```python
from build123d import *

# Parameters (mm, degrees)
SKETCH1_W           = 23.8
SKETCH1_H           = 9.8
BOSS_EXTRUDE1_DEPTH = 1
SKETCH2_W           = 3
SKETCH2_H           = 6.1
BOSS_EXTRUDE2_DEPTH = 3.25
SKETCH4_W           = 1
SKETCH4_H           = 6.1
BOSS_EXTRUDE3_DEPTH = 1
SKETCH3_R           = 3.3
CUT_EXTRUDE1_DEPTH  = 19.25
FILLET1_R           = 0.2


with BuildPart() as part:
    # Sketch1 → Boss-Extrude1 (new body)
    with BuildSketch(Plane(origin=(0, 0, 0), x_dir=(1, 0, 0), z_dir=(0, 1, 0))):
        with Locations((-11.9, 4.9)):
            Rectangle(SKETCH1_W, SKETCH1_H)
    extrude(amount=BOSS_EXTRUDE1_DEPTH)

    # Sketch2 → Boss-Extrude2 (add)
    with BuildSketch(Plane(origin=(0, 1, 0), x_dir=(1, 0, 0), z_dir=(0, 1, 0))):
        with Locations((-0.5, 5.65)):
            Rectangle(SKETCH2_W, SKETCH2_H)
    extrude(amount=BOSS_EXTRUDE2_DEPTH)

    # Sketch4 → Boss-Extrude3 (add)
    with BuildSketch(Plane.XZ.offset(-1)):
        with Locations((0.5, -5.65)):
            Rectangle(SKETCH4_W, SKETCH4_H)
    extrude(amount=BOSS_EXTRUDE3_DEPTH)

    # Sketch3 → Cut-Extrude1 (cut)
    with BuildSketch(Plane(origin=(1, 0, 0), x_dir=(0, 0, -1), z_dir=(1, 0, 0))):
        with Locations((5.65, 4.25)):
            Circle(SKETCH3_R)
    extrude(amount=-CUT_EXTRUDE1_DEPTH, mode=Mode.SUBTRACT)

    # Fillet1
    fillet1_edges = [part.edges().sort_by_distance(p)[0] for p in [
        (-0.5, 2.990039683, -2.6),
        (-0.5, 2.990039683, -8.7),
    ]]
    fillet(fillet1_edges, radius=FILLET1_R)


solid = part.part
```
Verification items for the finished model (mm, model axes). A direction names the side the tool comes from. Coordinates: 2 decimals unless noted, no trailing zeros. Loops run counter-clockwise (first coordinate to the right, second up) from the corner with the lowest first, then second, coordinate; pieces in that order, holes last. Notation, with made-up numbers: (9.5, -2.5) - (13.5, -2.5) arc R24 cw to (13.5, 20.5) - close; hole circle Ø6 at (87, -9). An arc over 180 degrees is marked (long way). Answer as a JSON object with one key per item and string values.
(1) Scan lines: line 1 along X through (y, z) = (2.35, -8.5); line 2 along Y through (x, z) = (-13.25, -1); line 3 along X through (y, z) = (0.2, -9). Record each from-to range of solid material in increasing order.
Response:
{"line 1": "x = -2 to 1", "line 2": "y = 0 to 1", "line 3": "x = -23.8 to 0"}
(2) Go/stop test with flat-tipped pins: pin 1 Ø1.1 at (y, z) = (2, -8) entering from -X; pin 2 Ø3 at (x, z) = (-15.5, -5) entering from +Y; pin 3 Ø0.8 at (y, z) = (0.5, -1) entering from +X. Record where each tip stops, or that it passes through.
Response:
{"pin 1": "stops at x = -2", "pin 2": "stops at y = 1", "pin 3": "stops at x = 0"}
(3) Cross-section at A-A, the plane y = 1.8. Record the boundary of the cut face in (x, z).
Response:
{"outline": "(-2, -8.7) - (1, -8.7) - (1, -7.86) - (-2, -7.86) - close; (-2, -3.44) - (1, -3.44) - (1, -2.6) - (-2, -2.6) - close"}
(4) Cross-section at D-D, the plane z = -1.75. Record the boundary of the cut face in (x, y), then the cut area to 3 significant figures.
Response:
{"outline": "(-23.8, 0) - (0, 0) - (0, 1) - (-23.8, 1) - close", "area": "23.8 mm²"}
(5) Cross-section at B-B, the plane x = -1. Record the boundary of the cut face in (y, z).
Response:
{"outline": "(0, -9.8) - (1, -9.8) - (1, -8.7) - (2.22, -8.7) arc R0.2 ccw to (2.33, -8.34) arc R3.3 cw to (2.33, -2.96) arc R0.2 ccw to (2.22, -2.6) - (1, -2.6) - (1, 0) - (0, 0) - close"}
(6) Cross-section at C-C, the plane y = 0.6. Record the boundary of the cut face in (x, z), then the cut area to 3 significant figures.
Response:
{"outline": "(-23.8, -9.8) - (0, -9.8) - (0, -8.7) - (1, -8.7) - (1, -2.6) - (0, -2.6) - (0, 0) - (-23.8, 0) - close", "area": "239 mm²"}
(7) Mould release check, pull along Z, two halves, no side actions. Record for faces 6 (the flat face through (-12, 1, -4)), 7 (the cylindrical face through (-5.02, 0.96, -5.4)), 8 (the flat face through (-12.1, 0.5, 0)), 9 (the flat face through (-12.1, 0.5, -9.8)): pulls with the +Z half, pulls with the -Z half, needs draft (parallel to the pull), parting line crosses it, or undercut.
Response:
{"face 6": "needs draft", "face 7": "undercut", "face 8": "pulls with the +Z half", "face 9": "pulls with the -Z half"}
(8) Access from +Z, -Z, +X, -X, +Y, -Y to the whole of each face (thin tool, end or side, straight path). Record for faces 1 (the flat face through (-23.8, 0.5, -4.8)), 2 (the flat face through (1, 0.7, -5.7)), 3 (the flat face through (-2, 1.5, -8)), 4 (the flat face through (0, 0.5, -9.2)), 5 (the flat face through (0, 0.5, -1.3)).
Response:
{"face 1": "+Z, -Z, -X, +Y, -Y", "face 2": "+Z, -Z, +X, +Y, -Y", "face 3": "+Z, -Z, -X, +Y", "face 4": "-Z, +X, +Y, -Y", "face 5": "+Z, +X, +Y, -Y"}
